Build history of the part. All positions in model axes, mm. Coordinates: 2 decimals unless noted, no trailing zeros. Loops run counter-clockwise (first coordinate to the right, second up) from the corner with the lowest first, then second, coordinate; pieces in that order, holes last.
Item 1: Drill centre lines: line 1 along Y through (x, z) = (37.5, 2.25); line 2 along Y through (x, z) = (-11.5, 1.6); line 3 along X through (y, z) = (23.5, 2.25). Where is each one in solid material? Low to high.
Item 2: Flat gauge pins, fed straight in: pin 1 (4 mm diameter, centred on x = 0, y = -20, fed in from -Z); pin 2 (0.6 mm diameter, centred on x = 10, z = 1, fed in from +Y). Where does each tip first touch, or does it go through?
Item 3: Cut at A-A (y = -23.5). List the corners of the cut face in (x, z), and give its area (3 significant figures).
Item 4: Cut at C-C (z = 1). Count the separate pieces of the cut face and the enclosed holes in it, and give its area (3 significant figures).
Item 5: Cut at B-B (x = -11.5). List the corners of the cut face in (y, z).
from build123d import *

# Parameters (mm, degrees)
F1_W     = 75
F1_H     = 64
F1_R     = 2.25
F2_DEPTH = 3
F3_R     = 5
F4_R     = 3
F5_DEPTH = 25
F6_W     = 10.5
F6_H     = 12.9868694071
F7_DEPTH = 25
F8_R     = 4.99999


# Not quite as in the source:
# - a fillet or chamfer is up to 0.001 mm smaller than in the source, because OpenCascade refuses the exact size


with BuildPart() as f2:
    # F1 (on Top) → F2 (new body)
    with BuildSketch(Plane.XY):
        with Locations((7, 0)):
            Rectangle(F1_W, F1_H)
        with Locations((0, -20)):
            Circle(F1_R, mode=Mode.SUBTRACT)
        with Locations((37.5, -20)):
            Circle(F1_R, mode=Mode.SUBTRACT)
        with Locations((0, 20)):
            Circle(F1_R, mode=Mode.SUBTRACT)
        with Locations((37.5, 20)):
            Circle(F1_R, mode=Mode.SUBTRACT)
    extrude(amount=F2_DEPTH)

    # F3
    f3_edges = [f2.edges().sort_by_distance(p)[0] for p in [
        (-30.5, 32, 1.5),
        (-30.5, -32, 1.5),
        (44.5, -32, 1.5),
        (44.5, 32, 1.5),
    ]]
    fillet(f3_edges, radius=F3_R)

    # F4 (on Top) → F5 (cut)
    with BuildSketch(Plane.XY):
        with Locations((25.5, 23.5)):
            Circle(F4_R)
        with Locations((-11.5, 23.5)):
            Circle(F4_R)
        with Locations((25.5, -23.5)):
            Circle(F4_R)
        with Locations((-11.5, -23.5)):
            Circle(F4_R)
    extrude(amount=F5_DEPTH, mode=Mode.SUBTRACT)

    # F6 (on Top) → F7 (cut)
    with BuildSketch(Plane.XY):
        with Locations((10.25, 28.4934347035)):
            Rectangle(F6_W, F6_H)
    extrude(amount=F7_DEPTH, mode=Mode.SUBTRACT)

    # F8 (radius 5 in the source; OpenCascade refuses exactly that, so slightly less here)
    f8_edges = [f2.edges().sort_by_distance(p)[0] for p in [
        (5, 32, 1.5),
        (5, 22, 1.5),
        (15.5, 32, 1.5),
        (15.5, 22, 1.5),
    ]]
    fillet(f8_edges, radius=F8_R)


solid = f2.part
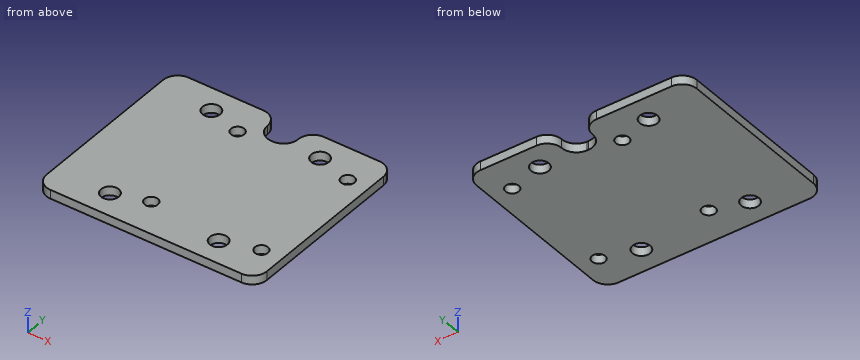
Filled sheet:
1. line 1: y = -32 to -22.25, -17.75 to 17.75, 22.25 to 32
1. line 2: y = -32 to -26.5, -20.5 to 20.5, 26.5 to 32
1. line 3: x = -30.5 to -14.5, -8.5 to 6.43, 14.07 to 22.5, 28.5 to 44.5
2. pin 1: passes through
2. pin 2: stops at y = 22.01
3. outline: (-30.5, 0) - (-14.5, 0) - (-14.5, 3) - (-30.5, 3) - close; (-8.5, 0) - (22.5, 0) - (22.5, 3) - (-8.5, 3) - close; (28.5, 0) - (44.5, 0) - (44.5, 3) - (28.5, 3) - close
3. area: 189 mm2
4. separate pieces: 1
4. enclosed holes: 8
4. area: 4,500 mm2
5. outline: (-32, 0) - (-26.5, 0) - (-26.5, 3) - (-32, 3) - close; (-20.5, 0) - (20.5, 0) - (20.5, 3) - (-20.5, 3) - close; (26.5, 0) - (32, 0) - (32, 3) - (26.5, 3) - close
